Check sheet for the modelled part. Datum: model origin and axes. Units: mm. A direction names the side the tool comes from. Coordinates: 2 decimals unless noted, no trailing zeros. Loops run counter-clockwise (first coordinate to the right, second up) from the corner with the lowest first, then second, coordinate; pieces in that order, holes last.
```python
from build123d import *

# Parameters (mm, degrees)
SKETCH_1_R      = 2.75
SKETCH_1_R_2    = 8
SKETCH_1_R_3    = 1.5
EXTRUDE_1_DEPTH = 5
CHAMFER_1_SIZE  = 2.5


with BuildPart() as part:
    # 草图1 → 拉伸1 (new body)
    with BuildSketch(Plane.XY):
        with BuildLine():
            Line((1708.420547593, 1108.565488817), (1708.420547593, 1091.565488817))
            Line((1708.420547593, 1091.565488817), (1727.920547593, 1065.065488817))
            Line((1727.920547593, 1065.065488817), (1727.920547593, 1040.065488817))
            Line((1727.920547593, 1040.065488817), (1716.420547593, 1040.065488817))
            ThreePointArc((1716.420547593, 1040.065488817), (1714.29922725, 1039.186809161), (1713.420547593, 1037.065488817))
            Line((1713.420547593, 1037.065488817), (1713.420547593, 1008.065488817))
            ThreePointArc((1713.420547593, 1008.065488817), (1714.29922725, 1005.944168474), (1716.420547593, 1005.065488817))
            Line((1716.420547593, 1005.065488817), (1745.420547593, 1005.065488817))
            ThreePointArc((1745.420547593, 1005.065488817), (1747.541867937, 1005.944168474), (1748.420547593, 1008.065488817))
            Line((1748.420547593, 1008.065488817), (1748.420547593, 1108.565488817))
            ThreePointArc((1748.420547593, 1108.565488817), (1747.541867937, 1110.686809161), (1745.420547593, 1111.565488817))
            Line((1745.420547593, 1111.565488817), (1711.420547593, 1111.565488817))
            ThreePointArc((1711.420547593, 1111.565488817), (1709.29922725, 1110.686809161), (1708.420547593, 1108.565488817))
        make_face()
        with Locations((1718.920547593, 1010.565488817)):
            Circle(SKETCH_1_R, mode=Mode.SUBTRACT)
        with Locations((1718.920547593, 1034.565488817)):
            Circle(SKETCH_1_R, mode=Mode.SUBTRACT)
        with Locations((1730.920547593, 1022.565488817)):
            Circle(SKETCH_1_R_2, mode=Mode.SUBTRACT)
        with Locations((1742.920547593, 1010.565488817)):
            Circle(SKETCH_1_R, mode=Mode.SUBTRACT)
        with Locations((1742.920547593, 1034.565488817)):
            Circle(SKETCH_1_R, mode=Mode.SUBTRACT)
        with Locations((1742.920547593, 1045.565488817)):
            Circle(SKETCH_1_R_3, mode=Mode.SUBTRACT)
        with Locations((1742.920547593, 1055.565488817)):
            Circle(SKETCH_1_R_3, mode=Mode.SUBTRACT)
        with BuildLine():
            Line((1715.420547593, 1106.565488817), (1719.420547593, 1106.565488817))
            ThreePointArc((1719.420547593, 1106.565488817), (1722.420547593, 1103.565488817), (1719.420547593, 1100.565488817))
            Line((1719.420547593, 1100.565488817), (1715.420547593, 1100.565488817))
            ThreePointArc((1715.420547593, 1100.565488817), (1712.420547593, 1103.565488817), (1715.420547593, 1106.565488817))
        make_face(mode=Mode.SUBTRACT)
        with BuildLine():
            ThreePointArc((1737.420547593, 1100.565488817), (1734.420547593, 1103.565488817), (1737.420547593, 1106.565488817))
            Line((1737.420547593, 1106.565488817), (1741.420547593, 1106.565488817))
            ThreePointArc((1741.420547593, 1106.565488817), (1744.420547593, 1103.565488817), (1741.420547593, 1100.565488817))
            Line((1741.420547593, 1100.565488817), (1737.420547593, 1100.565488817))
        make_face(mode=Mode.SUBTRACT)
    extrude(amount=EXTRUDE_1_DEPTH)

    # 倒角1
    chamfer_1_edges = [part.edges().sort_by_distance(p)[0] for p in [
        (1740.170547593, 1034.565488817, 0),
        (1740.170547593, 1010.565488817, 0),
        (1716.170547593, 1010.565488817, 0),
        (1716.170547593, 1034.565488817, 0),
    ]]
    chamfer(chamfer_1_edges, length=CHAMFER_1_SIZE)


solid = part.part
```
1) Section check A-A on y = 1102.5. Enter the section's corners in (x, z).
Answer sheet:
outline: (1708.42, 0) - (1712.62, 0) - (1712.62, 5) - (1708.42, 5) - close; (1722.22, 0) - (1734.62, 0) - (1734.62, 5) - (1722.22, 5) - close; (1744.22, 0) - (1748.42, 0) - (1748.42, 5) - (1744.22, 5) - close
2) Scan lines: line 1 (Y direction, x = 1743.5, z = 0.5); line 2 (Y direction, x = 1743, z = 2.25); line 3 (Y direction, x = 1721, z = 2.85). Record each from-to range of solid material in increasing order.
Answer sheet:
line 1: y = 1005.07 to 1005.85, 1015.28 to 1029.85, 1039.28 to 1044.18, 1046.95 to 1054.18, 1056.95 to 1101.4, 1105.73 to 1111.57
line 2: y = 1005.07 to 1007.57, 1013.56 to 1031.57, 1037.56 to 1044.07, 1047.06 to 1054.07, 1057.06 to 1101.01, 1106.12 to 1111.57
line 3: y = 1005.07 to 1008.77, 1012.37 to 1032.77, 1036.37 to 1040.07, 1074.47 to 1101.01, 1106.12 to 1111.57
3) Set-up check for faces 1 (the flat face through (1733, 1071, 0)), 2 (the flat face through (1727.921, 1053, 2)), 3 (the flat face through (1717, 1106.565, 2)): record each of +Z, -Z, +X, -X, +Y, -Y from which the full face is reachable in a straight line by a thin tool's end or side.
Answer sheet:
face 1: -Z, +X, -X, +Y, -Y
face 2: +Z, -Z, -X
face 3: +Z, -Z
4) Depth check by flat-ended pin: pin 1 (7 mm diameter, centred on x = 1742.92, y = 1034.57, fed in from -Z). Enter the tip coordinate at first touch or a pass-through.
Answer sheet:
pin 1: stops at z = 1.75
5) Section check C-C on x = 1730.5. Enter the section's corners in (y, z), plus the area to 3 significant figures.
Answer sheet:
outline: (1005.07, 0) - (1014.58, 0) - (1014.58, 5) - (1005.07, 5) - close; (1030.55, 0) - (1111.57, 0) - (1111.57, 5) - (1030.55, 5) - close
area: 453 mm2
6) Section check B-B on y = 1019.5. Enter the section's corners in (x, z), plus the area to 3 significant figures.
Answer sheet:
outline: (1713.42, 0) - (1723.53, 0) - (1723.53, 5) - (1713.42, 5) - close; (1738.31, 0) - (1748.42, 0) - (1748.42, 5) - (1738.31, 5) - close
area: 101 mm2
7) Mould release check, pull along X, two halves, no side actions. Record for faces 4 (the cylindrical face through (1714.276, 1005.968, 2.465)), 5 (the cylindrical face through (1747.52, 1005.92, 2.46)), 6 (the cylindrical face through (1734.42, 1103.5, 2.46)): +X half, -X half, draft (parallel to the pull), parting line (faces both ways), or undercut.
Answer sheet:
face 4: -X half
face 5: +X half
face 6: undercut
8) Section check D-D on z = 0.95. Give the number of separate pieces and of enclosed holes in the cut face, plus the area to 3 significant figures.
Answer sheet:
separate pieces: 1
enclosed holes: 9
area: 2,780 mm2
